Verification items for the finished model (mm, model axes). Face numbers are marked on the shaded views. A direction names the side the tool comes from. Round coordinates to 2 decimals unless told otherwise and drop trailing zeros. Order: outer loops, then holes, each group sorted by start corner. A loop starts at its lowest first (then second) coordinate and runs counter-clockwise, first axis right, second up. Notation, with made-up numbers: M 32.5,0.25 L 70.5,0.25 A8 cw 70.5,6.25 Z; hole C -17.5,44 d5. An arc over 180 degrees is marked long. Write item = value, one per line. Start each with the question number.
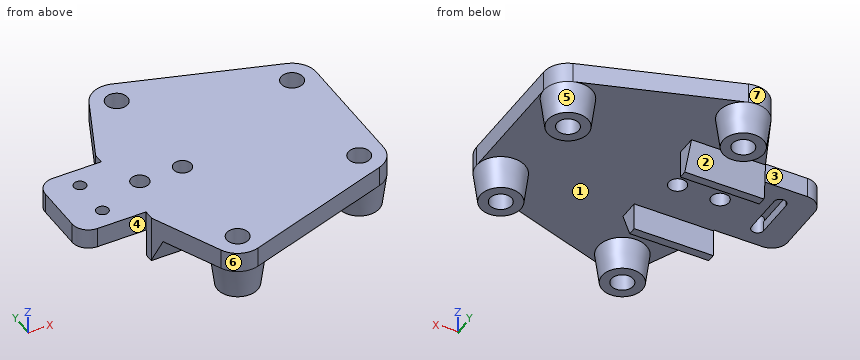
from build123d import *

# Parameters (mm, degrees)
SKETCH_1_R          = 2.2
SKETCH_1_R_2        = 2.7
SKETCH_1_R_3        = 1.5
EXTRUDE_1_DEPTH     = 5
SKETCH_1_4_W        = 19.5
SKETCH_1_4_H        = 2
EXTRUDE_2_DEPTH     = 6.8
CHAMFER_1_SIZE2     = 6.8
CHAMFER_1_SIZE      = 3
CHAMFER_2_SIZE2     = 6.8
CHAMFER_2_SIZE      = 3
CUT_EXTRUDE_1_DEPTH = 2.5


with BuildPart() as part:
    # 草图1 → 凸台-拉伸1 (new body)
    with BuildSketch(Plane.XY):
        with BuildLine():
            Line((-23.759975961, 29.487702254), (-31.5, 12.5))
            Line((-31.5, 12.5), (-31.5, 10))
            Line((-31.5, 10), (-43.5, 10))
            ThreePointArc((-43.5, 10), (-46.328427125, 8.828427125), (-47.5, 6))
            Line((-47.5, 6), (-47.5, -6))
            ThreePointArc((-47.5, -6), (-46.328427125, -8.828427125), (-43.5, -10))
            Line((-43.5, -10), (-31.5, -10))
            Line((-31.5, -10), (-31.5, -12.5))
            Line((-31.5, -12.5), (-23.759975961, -29.487702254))
            ThreePointArc((-23.759975961, -29.487702254), (-20.709389548, -32.494983349), (-16.430695985, -32.701377246))
            Line((-16.430695985, -32.701377246), (20.169304015, -20.701377246))
            ThreePointArc((20.169304015, -20.701377246), (23.158797387, -18.520239758), (24.3, -15))
            Line((24.3, -15), (24.3, 15))
            ThreePointArc((24.3, 15), (23.158797387, 18.520239758), (20.169304015, 20.701377246))
            Line((20.169304015, 20.701377246), (-16.430695985, 32.701377246))
            ThreePointArc((-16.430695985, 32.701377246), (-20.709389548, 32.494983349), (-23.759975961, 29.487702254))
        make_face()
        with Locations((-17, 0)):
            Circle(SKETCH_1_R, mode=Mode.SUBTRACT)
        with Locations((-27.5, 0)):
            Circle(SKETCH_1_R, mode=Mode.SUBTRACT)
        with Locations((18.3, 15)):
            Circle(SKETCH_1_R_2, mode=Mode.SUBTRACT)
        with Locations((-39.5, 5)):
            Circle(SKETCH_1_R_3, mode=Mode.SUBTRACT)
        with Locations((-39.5, -5)):
            Circle(SKETCH_1_R_3, mode=Mode.SUBTRACT)
        with Locations((18.3, -15)):
            Circle(SKETCH_1_R_2, mode=Mode.SUBTRACT)
        with Locations((-18.3, 27)):
            Circle(SKETCH_1_R_2, mode=Mode.SUBTRACT)
        with Locations((-18.3, -27)):
            Circle(SKETCH_1_R_2, mode=Mode.SUBTRACT)
    extrude(amount=EXTRUDE_1_DEPTH)

    # 草图4 → 旋转1 (revolve)
    with BuildSketch(Plane(origin=(6.216937636, 18.961659791, 0), x_dir=(-0.9502295409734977, 0.31155066917163887, 0), z_dir=(-0.31155066917163887, -0.9502295409734977, 0)), mode=Mode.PRIVATE) as revolve_1_sk:
        Polygon((-6.715940562, 0), (-7.715940562, 7.7), (-10.015940562, 7.7), (-10.015940562, 0), align=None)
    revolve_1 = revolve(revolve_1_sk.sketch.rotate(Axis((18.3, 15, 4.45283877), (0, 0, -1)), 161.847294113), axis=Axis((18.3, 15, 4.45283877), (0, 0, -1)))

    # 草图4<3> → 旋转2 (revolve)
    with BuildSketch(Plane(origin=(6.216937636, 18.961659791, 0), x_dir=(-0.9502295409734977, 0.31155066917163887, 0), z_dir=(-0.31155066917163887, -0.9502295409734977, 0)), mode=Mode.PRIVATE) as revolve_2_sk:
        Polygon((30.801068667, 7.7), (28.501068667, 7.7), (28.501068667, 0), (31.801068667, 0), align=None)
    revolve_2 = revolve(revolve_2_sk.sketch.rotate(Axis((-18.3, 27, 0), (0, 0, -1)), 161.847294113), axis=Axis((-18.3, 27, 0), (0, 0, -1)))

    # 镜向1: 旋转1, 旋转2 across plane
    add(revolve_1.mirror(Plane.ZX))
    add(revolve_2.mirror(Plane.ZX))

    # 草图1<4> → 凸台-拉伸2 (add)
    with BuildSketch(Plane.XY):
        with Locations((-21.75, 11.3)):
            Rectangle(SKETCH_1_4_W, SKETCH_1_4_H)
        with Locations((-21.75, -11.3)):
            Rectangle(SKETCH_1_4_W, SKETCH_1_4_H)
    extrude(amount=-EXTRUDE_2_DEPTH)

    # 倒角1
    chamfer_1_edges = [part.edges().sort_by_distance(p)[0] for p in [
        (-21.75, 12.3, 0),
    ]]
    chamfer_1_side = [part.faces().sort_by_distance(p)[0] for p in [
        (-21.75, 12.36, 0),
    ]]
    chamfer(chamfer_1_edges, length=CHAMFER_1_SIZE - 0.0001, length2=CHAMFER_1_SIZE2 - 0.0001, reference=chamfer_1_side[0])  # a hair under: the kernel refuses the full size

    # 倒角2
    chamfer_2_edges = [part.edges().sort_by_distance(p)[0] for p in [
        (-21.75, -12.3, 0),
    ]]
    chamfer_2_side = [part.faces().sort_by_distance(p)[0] for p in [
        (-21.75, -12.36, 0),
    ]]
    chamfer(chamfer_2_edges, length=CHAMFER_2_SIZE - 0.0001, length2=CHAMFER_2_SIZE2 - 0.0001, reference=chamfer_2_side[0])  # a hair under: the kernel refuses the full size

    # 草图5 → 切除-拉伸1 (cut)
    with BuildSketch(Plane(origin=(0, 0, 0), x_dir=(-1, 0, 0), z_dir=(0, 0, -1))):
        with BuildLine():
            Line((41, 5), (41, -5))
            ThreePointArc((41, -5), (39.5, -6.5), (38, -5))
            Line((38, -5), (38, 5))
            ThreePointArc((38, 5), (39.5, 6.5), (41, 5))
        make_face()
    extrude(amount=-CUT_EXTRUDE_1_DEPTH, mode=Mode.SUBTRACT)


solid = part.part
1) Scan lines: probe 1 along Y at (x, z) = (-39.5, 1.25); probe 2 along Z at (x, y) = (-2, -5.5); probe 3 along Y at (x, z) = (-14, -2.5). Record each from-to range of solid material in increasing order.
2) Access from +Z, -Z, +X, -X, +Y, -Y to the whole of each face (thin tool, end or side, straight path). Record for the marked faces 1, 2, 3 and 4.
3) Gauge pin test, flat ends, axial feed: P1, Ø5.5, axis at x = -27.5, y = 0, coming from the -Z side; P2, Ø5.5, axis at x = -19, z = -4.5, coming from the +Y side; P3, Ø1, axis at x = -22, y = 11, coming from the -Z side; P4, Ø5, axis at y = -2, z = -0.5, coming from the +X side. Record the tip position at first contact, or that the pin passes through.
4) Cross-section at C-C, the plane x = 18.3. Enter the section's corners in (y, z), then the cut area to 3 significant figures.
5) Cross-section at B-B, the plane y = 0. Enter the section's corners in (x, z), then the cut area to 4 significant figures.
6) Cross-section at A-A, the plane z = -2.5. Give the number of separate pieces and of enclosed holes in the cut face, then the cut area to 3 significant figures.
7) Release check for a two-part mould opening along Y. For the marked faces 5, 6 and 7 record: pulls with the +Y half, pulls with the -Y half, needs draft (parallel to the pull), parting line crosses it, or undercut.
Geometry results:
q1.probe_1 = -10 to -6.5, 6.5 to 10
q1.probe_2 = 0 to 5
q1.probe_3 = -30.7 to -23.3, -14.2 to -10.3, 10.3 to 14.2, 23.3 to 30.7
q2.face_1 = -Z
q2.face_2 = -Z, -X
q2.face_3 = +Z, -Z, -X, +Y
q2.face_4 = +Z, -Z, -X, -Y
q3.P1 = 0
q3.P2 = 32.76
q3.P3 = -6.8
q3.P4 = 24.3
q4.outline = M -21.31,0 L -21,0 L -20,-7.7 L -17.7,-7.7 L -17.7,5 L -21.31,5 Z; M -12.3,-7.7 L -10,-7.7 L -9,0 L 9,0 L 10,-7.7 L 12.3,-7.7 L 12.3,5 L -12.3,5 Z; M 17.7,-7.7 L 20,-7.7 L 21,0 L 21.31,0 L 21.31,5 L 17.7,5 Z
q4.area = 245 mm^2
q5.outline = M -47.5,0 L -41,0 L -41,2.5 L -38,2.5 L -38,0 L -29.7,0 L -29.7,5 L -47.5,5 Z; M -25.3,0 L -19.2,0 L -19.2,5 L -25.3,5 Z; M -14.8,0 L 24.3,0 L 24.3,5 L -14.8,5 Z
q5.area = 307.5 mm^2
q6.separate_pieces = 6
q6.enclosed_holes = 4
q6.area = 464 mm^2
q7.face_5 = undercut
q7.face_6 = pulls with the -Y half
q7.face_7 = pulls with the +Y half
